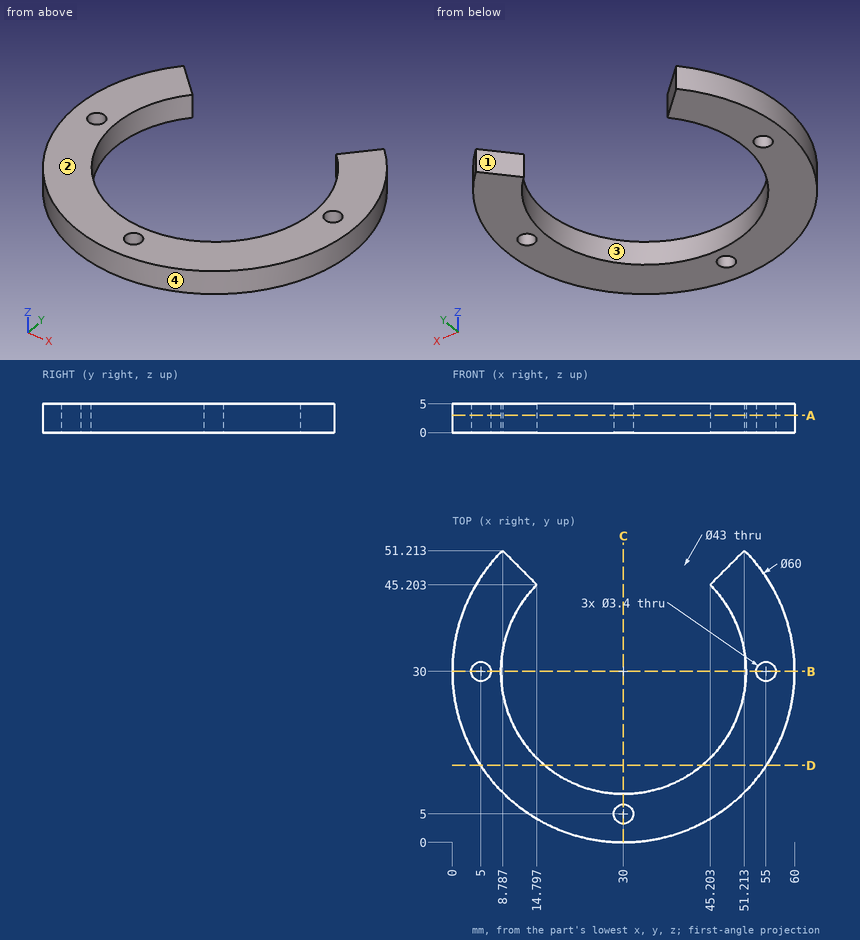
Can you work these out from the drawing? Everything is in mm from the part's minimum corner. Give positions to 0.01 mm unless a question says otherwise; leave off trailing zeros. Order: outer loops, then holes, each group sorted by start corner. A loop starts at its lowest first (then second) coordinate and runs counter-clockwise, first axis right, second up.
1. Suppose I cut it at D-D (y = 13.5). List the corners of the cut face in (x, z) for me (3 decimals).
2. Suppose I cut it at B-B (y = 30). List the corners of the cut face in (x, z) for me.
3. Will this pin go through, and if not, where does the flat tip stop? P1, Ø2, axis at x = 47, z = 4, coming from the +Y side.
4. I need wall thicknesses on L1, parallel to X at y = 19.5, z = 2; L2, parallel to Y at x = 3.5, z = 4.6; L3, parallel to Y at x = 5, z = 3.9. Which ranges of each line are inside material? Lowest first, please.
5. Suppose I cut it at A-A (z = 3). List the corners of the cut face in (x, y) for me, plus the area to 3 significant figures.
6. We'd pull the mould along X, two halves only. Please class the marked faces 1, 2, 3 and 4: pulls with the +X half, pulls with the -X half, needs draft (parallel to the pull), parting line crosses it, or undercut.
7. Suppose I cut it at C-C (x = 30). List the corners of the cut face in (y, z) for me.
Solved:
1. outline: (4.945, 0) - (16.216, 0) - (16.216, 5) - (4.945, 5) - close; (43.784, 0) - (55.055, 0) - (55.055, 5) - (43.784, 5) - close
2. outline: (0, 0) - (3.3, 0) - (3.3, 5) - (0, 5) - close; (6.7, 0) - (8.5, 0) - (8.5, 5) - (6.7, 5) - close; (51.5, 0) - (53.3, 0) - (53.3, 5) - (51.5, 5) - close; (56.7, 0) - (60, 0) - (60, 5) - (56.7, 5) - close
3. P1: stops at y = 48
4. L1: x = 1.9 to 11.24, 48.76 to 58.1
4. L2: y = 15.94 to 29.2, 30.8 to 44.06
4. L3: y = 13.42 to 28.3, 31.7 to 46.58
5. outline: (8.79, 51.21) arc R30 ccw (long way) to (51.21, 51.21) - (45.2, 45.2) arc R21.5 cw (long way) to (14.8, 45.2) - close; hole circle Ø3.4 at (5, 30); hole circle Ø3.4 at (30, 5); hole circle Ø3.4 at (55, 30)
5. area: 1,000 mm2
6. face 1: undercut
6. face 2: needs draft
6. face 3: undercut
6. face 4: parting line crosses it
7. outline: (0, 0) - (3.3, 0) - (3.3, 5) - (0, 5) - close; (6.7, 0) - (8.5, 0) - (8.5, 5) - (6.7, 5) - close
